Model file for the job. Use its own axes, mm. A direction names the side the tool comes from. Round coordinates to 2 decimals unless told otherwise and drop trailing zeros. Loops run counter-clockwise (first coordinate to the right, second up) from the corner with the lowest first, then second, coordinate; pieces in that order, holes last. Notation, with made-up numbers: (64.25, 83.5) - (86.25, 83.5) arc R11 ccw to (86.25, 103.5) - close; hole circle Ø10 at (87.25, 39.5). An arc over 180 degrees is marked (long way). Answer as a JSON object with one key per item and string values.
from build123d import *

# Parameters (mm, degrees)
SKETCH1_R           = 16
BOSS_EXTRUDE1_DEPTH = 10
SKETCH2_W           = 22
SKETCH2_H           = 22
BOSS_EXTRUDE2_DEPTH = 5
SKETCH3_R           = 9.75
CUT_EXTRUDE1_DEPTH  = 28.147743921
FILLET1_R           = 3


with BuildPart() as part:
    # Sketch1 → Boss-Extrude1 (new body)
    with BuildSketch(Plane(origin=(0, 0, 0), x_dir=(1, 0, 0), z_dir=(0, 1, 0))):
        with Locations(Location((0, 0, 0), (0, 0, 270))):
            Circle(SKETCH1_R)
    extrude(amount=BOSS_EXTRUDE1_DEPTH)

    # Sketch2 → Boss-Extrude2 (add)
    with BuildSketch(Plane.XZ):
        Rectangle(SKETCH2_W, SKETCH2_H)
    extrude(amount=BOSS_EXTRUDE2_DEPTH)

    # Sketch3 → Cut-Extrude1 (cut, through all)
    with BuildSketch(Plane(origin=(0, 10, 0), x_dir=(1, 0, 0), z_dir=(0, 1, 0))):
        with Locations(Location((0, 0, 0), (0, 0, 270))):
            Circle(SKETCH3_R)
    extrude(amount=-CUT_EXTRUDE1_DEPTH, mode=Mode.SUBTRACT)

    # Fillet1
    fillet1_edges = [part.edges().sort_by_distance(p)[0] for p in [
        (0, 10, -16),
    ]]
    fillet(fillet1_edges, radius=FILLET1_R)


solid = part.part
1) Two-plate mould, pull along X, no slides. Class faces 1 (the flat face through (-10, -5, 0)), 2 (the cylindrical face through (-15.62, 3.45, -3.47)), 3 (the cylindrical face through (9.667, 2.605, -1.269)): pulls with the +X half, pulls with the -X half, needs draft (parallel to the pull), parting line crosses it, or undercut.
Values follow:
{"face 1": "needs draft", "face 2": "parting line crosses it", "face 3": "undercut"}
2) Slice it at B-B on x = 0. List the corners of the cut face in (y, z).
Values follow:
{"outline": "(-5, -11) - (0, -11) - (0, -16) - (7, -16) arc R3 ccw to (10, -13) - (10, -9.75) - (-5, -9.75) - close; (-5, 9.75) - (10, 9.75) - (10, 13) arc R3 ccw to (7, 16) - (0, 16) - (0, 11) - (-5, 11) - close"}
3) Slice it at A-A on z = 0. List the corners of the cut face in (x, y), then the cut area to 3 significant figures.
Values follow:
{"outline": "(-16, 0) - (-11, 0) - (-11, -5) - (-9.75, -5) - (-9.75, 10) - (-13, 10) arc R3 ccw to (-16, 7) - close; (9.75, -5) - (11, -5) - (11, 0) - (16, 0) - (16, 7) arc R3 ccw to (13, 10) - (9.75, 10) - close", "area": "134 mm²"}
4) Probe probe 1 along X at (y, z) = (1, 0); probe 2 along X at (y, z) = (-3.75, 10.5); probe 3 along X at (y, z) = (9.25, -3.5). List the from-to ranges inside material, lowest first.
Values follow:
{"probe 1": "-16 to -9.75, 9.75 to 16", "probe 2": "-11 to 11", "probe 3": "-14.57 to -9.1, 9.1 to 14.57"}
5) Drop flat-ended pins along their axis: P1, Ø6, axis at x = -3.5, y = 6.5, coming from the +Z side; P2, Ø1.5, axis at x = -1.5, y = -3, coming from the -Z side; P3, Ø4, axis at y = -1.5, z = -5, coming from the +X side. Give the stop position or say it passes through.
Values follow:
{"P1": "z = 15.99", "P2": "z = -11", "P3": "x = 15.57"}
6) Slice it at C-C on y = 2. List the corners of the cut face in (x, z).
Values follow:
{"outline": "circle Ø32 at (0, 0); hole circle Ø19.5 at (0, 0)"}
7) Tool access for faces 4 (the flat face through (10, 10, 2)), 5 (the flat face through (0, -2, -11)), 6 (the flat face through (0, -2, 11)), 7 (the flat face through (11, -2, 0)), 8 (the flat face through (-11, -2, 0)): list every direction of +Z, -Z, +X, -X, +Y, -Y with a clear straight run to the whole face (end or side of a thin tool).
Values follow:
{"face 4": "+Z, -Z, +X, -X, +Y", "face 5": "-Z, +X, -X, -Y", "face 6": "+Z, +X, -X, -Y", "face 7": "+Z, -Z, +X, -Y", "face 8": "+Z, -Z, -X, -Y"}
